Build history of the part. All positions in model axes, mm. A direction names the side the tool comes from. Give positions to 0.01 mm unless a question says otherwise; leave off trailing zeros. Order: outer loops, then holes, each group sorted by start corner. A loop starts at its lowest first (then second) coordinate and runs counter-clockwise, first axis right, second up. Notation, with made-up numbers: (-6, 54.25) - (16, 54.25) arc R16 ccw to (16, 65.25) - close; hole circle Ø2 at (25.5, 18). An arc over 180 degrees is marked (long way). Use a Markdown table: item, result. Add a question column.
(1) Wall check: line 1 (Y direction, x = 8585, z = 6); line 2 (Y direction, x = 8593.5, z = 1.5); line 3 (X direction, y = 2931, z = 5.5). Give the ranges that are in metal, low to high.
(2) Slice it at A-A (x = 8595). Write the cut outline in (y, z), then the cut area to 3 significant figures.
(3) Flat gauge pins, fed straight in: pin 1 (3 mm diameter, centred on x = 8651.5, z = 4.5, fed in from -Y); pin 2 (3 mm diameter, centred on x = 8657.5, z = 3.5, fed in from +Y); pin 3 (3.5 mm diameter, centred on y = 3012, z = 4.5, fed in from -X). Where does each tip first touch, or does it go through?
(4) Slice it at B-B (y = 2932). Write the cut outline in (x, z), then the cut area to 3 significant figures.
(5) Mould opens along Y. For faces 5 (the face through (8660.063, 2910.317, 3.131)), 6 (the face through (8662.207, 2957, 3)), 7 (the face through (8652.047, 2932, 3)) say: +Y half, -Y half, draft (parallel to the pull), parting line (faces both ways), or undercut.
(6) Which spindle directions (+Z, -Z, +X, -X, +Y, -Y) get a long thin tool onto all of the face, cutting with end or side? Do faces 1 (the face through (8590.39, 2973.82, 3.13)), 2 (the face through (8641.989, 3013, 3)), 3 (the face through (8649.507, 2998, 3)), 4 (the face through (8648, 2911.459, 3)). Say none if no direction does.
from build123d import *

# Parameters (mm, degrees)
BOSS_EXTRUDE1_DEPTH = 6.35


with BuildPart() as part:
    # Sketch1 → Boss-Extrude1 (new body)
    with BuildSketch(Plane.XY):
        with BuildLine():
            Line((8662.207393671, 3006.696553149), (8662.207393671, 3000.166824887))
            Line((8662.207393671, 3000.166824887), (8649.507393671, 3000.166824887))
            Line((8649.507393671, 3000.166824887), (8649.507393671, 2996.763224887))
            Line((8649.507393671, 2996.763224887), (8662.207393671, 2996.763224887))
            Line((8662.207393671, 2996.763224887), (8662.207393671, 2988.787624887))
            Line((8662.207393671, 2988.787624887), (8655.222393671, 2988.787624887))
            ThreePointArc((8655.222393671, 2988.787624887), (8652.977329641, 2987.857688918), (8652.047393671, 2985.612624887))
            Line((8652.047393671, 2985.612624887), (8652.047393671, 2976.087624887))
            ThreePointArc((8652.047393671, 2976.087624887), (8652.977329641, 2973.842560857), (8655.222393671, 2972.912624887))
            Line((8655.222393671, 2972.912624887), (8662.207393671, 2972.912624887))
            Line((8662.207393671, 2972.912624887), (8662.207393671, 2939.653253149))
            Line((8662.207393671, 2939.653253149), (8655.222393671, 2939.653253149))
            ThreePointArc((8655.222393671, 2939.653253149), (8652.977329641, 2938.723317179), (8652.047393671, 2936.478253149))
            Line((8652.047393671, 2936.478253149), (8652.047393671, 2926.953253149))
            ThreePointArc((8652.047393671, 2926.953253149), (8652.977329641, 2924.708189118), (8655.222393671, 2923.778253149))
            Line((8655.222393671, 2923.778253149), (8662.207393671, 2923.778253149))
            Line((8662.207393671, 2923.778253149), (8662.207393671, 2915.574053149))
            ThreePointArc((8662.207393671, 2915.574053149), (8660.005305295, 2910.257741525), (8654.688993671, 2908.055653149))
            Line((8654.688993671, 2908.055653149), (8654.688993671, 2911.459253149))
            Line((8654.688993671, 2911.459253149), (8641.988993671, 2911.459253149))
            Line((8641.988993671, 2911.459253149), (8641.988993671, 2908.055653149))
            Line((8641.988993671, 2908.055653149), (8601.399793671, 2908.055653149))
            Line((8601.399793671, 2908.055653149), (8601.399793671, 2911.459253149))
            Line((8601.399793671, 2911.459253149), (8588.699793671, 2911.459253149))
            Line((8588.699793671, 2911.459253149), (8588.699793671, 2908.055653149))
            ThreePointArc((8588.699793671, 2908.055653149), (8583.383482047, 2910.257741525), (8581.181393671, 2915.574053149))
            Line((8581.181393671, 2915.574053149), (8581.181393671, 2923.778253149))
            Line((8581.181393671, 2923.778253149), (8588.166393671, 2923.778253149))
            ThreePointArc((8588.166393671, 2923.778253149), (8590.411457701, 2924.708189118), (8591.341393671, 2926.953253149))
            Line((8591.341393671, 2926.953253149), (8591.341393671, 2936.478253149))
            ThreePointArc((8591.341393671, 2936.478253149), (8590.411457701, 2938.723317179), (8588.166393671, 2939.653253149))
            Line((8588.166393671, 2939.653253149), (8581.181393671, 2939.653253149))
            Line((8581.181393671, 2939.653253149), (8581.181393671, 2972.912624887))
            Line((8581.181393671, 2972.912624887), (8588.166393671, 2972.912624887))
            ThreePointArc((8588.166393671, 2972.912624887), (8590.411457701, 2973.842560857), (8591.341393671, 2976.087624887))
            Line((8591.341393671, 2976.087624887), (8591.341393671, 2985.612624887))
            ThreePointArc((8591.341393671, 2985.612624887), (8590.411457701, 2987.857688918), (8588.166393671, 2988.787624887))
            Line((8588.166393671, 2988.787624887), (8581.181393671, 2988.787624887))
            Line((8581.181393671, 2988.787624887), (8581.181393671, 2996.763224887))
            Line((8581.181393671, 2996.763224887), (8593.881393671, 2996.763224887))
            Line((8593.881393671, 2996.763224887), (8593.881393671, 3000.166824887))
            Line((8593.881393671, 3000.166824887), (8581.181393671, 3000.166824887))
            Line((8581.181393671, 3000.166824887), (8581.181393671, 3006.696553149))
            ThreePointArc((8581.181393671, 3006.696553149), (8583.383482047, 3012.012864772), (8588.699793671, 3014.214953149))
            Line((8588.699793671, 3014.214953149), (8588.699793671, 3010.811353149))
            Line((8588.699793671, 3010.811353149), (8601.399793671, 3010.811353149))
            Line((8601.399793671, 3010.811353149), (8601.399793671, 3014.214953149))
            Line((8601.399793671, 3014.214953149), (8641.988993671, 3014.214953149))
            Line((8641.988993671, 3014.214953149), (8641.988993671, 3010.811353149))
            Line((8641.988993671, 3010.811353149), (8654.688993671, 3010.811353149))
            Line((8654.688993671, 3010.811353149), (8654.688993671, 3014.214953149))
            ThreePointArc((8654.688993671, 3014.214953149), (8660.005305295, 3012.012864772), (8662.207393671, 3006.696553149))
        make_face()
    extrude(amount=BOSS_EXTRUDE1_DEPTH)


solid = part.part
Solution:
| question | item | result |
|---|---|---|
| 1 | line 1 | 2909.03 to 2923.78, 2939.65 to 2972.91, 2988.79 to 2996.76, 3000.17 to 3013.24 |
| 1 | line 2 | 2911.46 to 2996.76, 3000.17 to 3010.81 |
| 1 | line 3 | 8591.34 to 8652.05 |
| 2 | outline | (2911.46, 0) - (3010.81, 0) - (3010.81, 6.35) - (2911.46, 6.35) - close |
| 2 | area | 631 mm2 |
| 3 | pin 1 | y = 2911.46 |
| 3 | pin 2 | y = 3014.1 |
| 3 | pin 3 | x = 8582.07 |
| 4 | outline | (8591.34, 0) - (8652.05, 0) - (8652.05, 6.35) - (8591.34, 6.35) - close |
| 4 | area | 385 mm2 |
| 5 | face 5 | -Y half |
| 5 | face 6 | draft |
| 5 | face 7 | undercut |
| 6 | face 1 | +Z, -Z, -X |
| 6 | face 2 | +Z, -Z, +Y |
| 6 | face 3 | +Z, -Z, +X |
| 6 | face 4 | +Z, -Z, -Y |
